Verification items for this drawing (mm, ordinates from the low corner). A direction names the side the tool comes from. Round coordinates to 2 decimals unless told otherwise and drop trailing zeros. Write each loop counter-clockwise with the first axis right and the second up, starting at its lowest first coordinate (ties: lowest second). Pieces come first, ordered by that corner, then holes.
Item 1: Access from +Z, -Z, +X, -X, +Y, -Y to the whole of each face (thin tool, end or side, straight path). Record for the marked faces 1, 2 and 3.
Item 2: Scan lines: probe 1 along Y at (x, z) = (15.1, 1.15); probe 2 along Y at (x, z) = (8.5, 6.25); probe 3 along Z at (x, y) = (17.75, 21). Record each from-to range of solid material in increasing order.
Item 3: Depth check by flat-ended pin: P1, Ø2, axis at x = 17, y = 24.5, coming from the +Z side; P2, Ø1, axis at y = 7.5, z = 1.5, coming from the -X side; P3, Ø4, axis at y = 10, z = 7, coming from the -X side. Enter the tip coordinate at first touch or a pass-through.
Item 4: Cross-section at C-C (x = 5.75). Enter the section's corners in (y, z), then the cut area to 3 significant figures.
Item 5: Cross-section at B-B (y = 8). Enter the section's corners in (x, z).
Item 6: Cross-section at A-A (z = 4.6). Enter the section's corners in (x, y), then the cut area to 3 significant figures.
Item 7: Draft check along X on the marked faces 4, 5 and 6. Enter one of: pulls with the +X half, pulls with the -X half, needs draft (parallel to the pull), parting line crosses it, or undercut.
Item 8: Cross-section at D-D (z = 8.75). Enter the section's corners in (x, y).
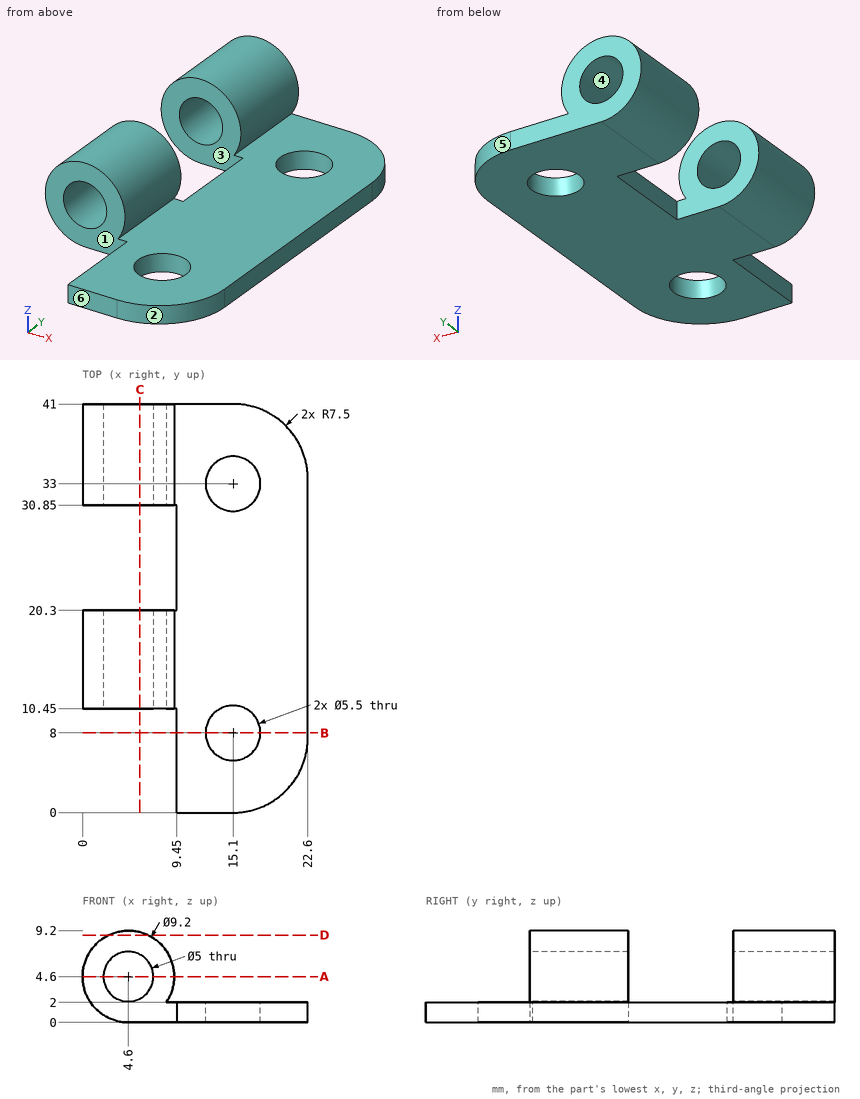
Resolved:
1. face 1: +Z, -Z, -X, -Y
1. face 2: +Z, -Z, +X, -Y
1. face 3: +Z, -Z, -X
2. probe 1: y = 0 to 5.25, 10.75 to 30.25, 35.75 to 41
2. probe 2: y = 10.45 to 20.3, 30.85 to 41
2. probe 3: z = 0 to 2
3. P1: stops at z = 2
3. P2: stops at x = 9.45
3. P3: stops at x = 0.02
4. outline: (10.45, 0) - (20.3, 0) - (20.3, 2.38) - (10.45, 2.38) - close; (10.45, 6.82) - (20.3, 6.82) - (20.3, 9.05) - (10.45, 9.05) - close; (30.85, 0) - (41, 0) - (41, 2.38) - (30.85, 2.38) - close; (30.85, 6.82) - (41, 6.82) - (41, 9.05) - (30.85, 9.05) - close
4. area: 92.3 mm2
5. outline: (9.45, 0) - (12.35, 0) - (12.35, 2) - (9.45, 2) - close; (17.85, 0) - (22.6, 0) - (22.6, 2) - (17.85, 2) - close
6. outline: (0, 10.45) - (2.1, 10.45) - (2.1, 20.3) - (0, 20.3) - close; (0, 30.85) - (2.1, 30.85) - (2.1, 41) - (0, 41) - close; (7.1, 10.45) - (9.2, 10.45) - (9.2, 20.3) - (7.1, 20.3) - close; (7.1, 30.85) - (9.2, 30.85) - (9.2, 41) - (7.1, 41) - close
6. area: 84.0 mm2
7. face 4: undercut
7. face 5: pulls with the +X half
7. face 6: needs draft
8. outline: (2.62, 10.45) - (6.58, 10.45) - (6.58, 20.3) - (2.62, 20.3) - close; (2.62, 30.85) - (6.58, 30.85) - (6.58, 41) - (2.62, 41) - close
